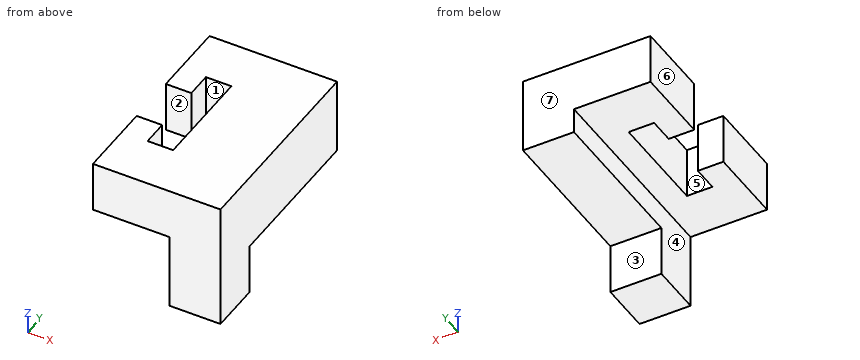
Autodesk Inventor part; units mm, degrees
ref_plane "YZ Plane" through (0, 0, 0) normal (1, 0, 0) x (0, 1, 0)
ref_plane "XZ Plane" through (0, 0, 0) normal (0, 1, 0) x (-1, 0, 0)
ref_plane "XY Plane" through (0, 0, 0) normal (0, 0, 1) x (1, 0, 0)
sketch "Náčrt1" plane through (0, 0, 0) normal (1, 0, 0) x (0, 1, 0)
  line L0 (0, 0) -> (0, -50)
  line L1 (0, -50) -> (80, -50)
  line L2 (80, -50) -> (80, 0)
  line L3 (80, 0) -> (0, 0)
  dimension "d0" = 50
  dimension "d1" = 80
extrude "Vysunutí1" add sketch "Náčrt1" along normal blind 50
sketch "Náčrt2" plane through (0, 0, -50) normal (0, 0, -1) x (-1, 0, 0)
  line L0 (-50, 0) -> (-50, 80)
  line L1 (-50, 0) -> (-50, 20)
  line L2 (-50, 20) -> (-30, 20)
  line L3 (-30, 20) -> (-30, 0)
  line L4 (0, 0) -> (-50, 0)
  line L5 (-30, 0) -> (-50, 0)
  line L6 (-50, 0) -> (-50, 80)
  line L7 (-50, 80) -> (-30, 80)
  line L8 (0, 80) -> (-50, 80)
  line L9 (-30, 80) -> (-30, 20)
  dimension "d4" = 20
  dimension "d5" = 20
  dimension "d6" = 20
extrude "Vysunutí2" cut sketch "Náčrt2" against normal blind 20 contours L0 L7 L9 L2
sketch "Náčrt3" plane through (0, 0, -50) normal (0, 0, -1) x (-1, 0, 0)
  line L0 (0, 80) -> (-50, 80)
  line L1 (0, 0) -> (0, 80)
  line L2 (0, 80) -> (0, 0)
  line L3 (0, 0) -> (-30, 0)
  line L4 (0, 0) -> (-50, 0)
  line L5 (-30, 0) -> (-30, 80)
  dimension "d9" = 30
extrude "Vysunutí3" cut sketch "Náčrt3" against normal blind 30
sketch "Náčrt4" plane through (0, 0, -20) normal (0, 0, -1) x (-1, 0, 0)
  line L0 (0, 80) -> (0, 0)
  line L1 (0, 40) -> (0, 30)
  line L2 (0, 30) -> (0, 50)
  line L3 (0, 50) -> (-10, 50)
  line L4 (0, 40) -> (-20, 40)
  line L5 (-20, 40) -> (-20, 60)
  line L6 (-20, 60) -> (-10, 60)
  line L7 (-10, 50) -> (-10, 60)
  line L8 (0, 30) -> (-10, 30)
  dimension "d12" = 10
  dimension "d13" = 20
  dimension "d14" = 10
  dimension "d15" = 20
  dimension "d16" = 20
  dimension "d17" = 10
extrude "Vysunutí4" cut sketch "Náčrt4" against normal blind 30
sketch "Náčrt5" plane through (0, 0, -20) normal (0, 0, -1) x (-1, 0, 0)
  line L0 (0, 40) -> (0, 0)
  line L1 (-20, 40) -> (-20, 60)
  line L2 (0, 40) -> (-20, 40)
  line L3 (-20, 40) -> (-20, 20)
  line L4 (-20, 20) -> (-10, 20)
  line L5 (-10, 20) -> (-10, 30)
  line L6 (-10, 30) -> (0, 30)
  line L7 (0, 40) -> (0, 0)
  line L8 (0, 30) -> (0, 40)
  dimension "d20" = 20
  dimension "d21" = 10
  dimension "d22" = 10
extrude "Vysunutí5" cut sketch "Náčrt5" against normal blind 30
properties part number "Martin-Probst-26673_obrazek_2"
Read the model definition and answer for the solid it produces. Units are mm, in the model's axes. Face numbers are marked on the shaded views. A direction names the side the tool comes from. Coordinates: 2 decimals unless noted, no trailing zeros. Write each loop counter-clockwise with the first axis right and the second up, starting at its lowest first coordinate (ties: lowest second). Pieces come first, ordered by that corner, then holes. Notation, with made-up numbers: M 52,0.5 L 91,0.5 A29 ccw 91,29.5 Z; hole C 70,-29.75 d11. An arc over 180 degrees is marked long. Use a Markdown table: item, result.
Q1. The part is cut by section B-B, the plane y = 58.5. Write down the section's boundary in (x, z), then the cut area to 3 significant figures.
Answer block:
| item | result |
|---|---|
| outline | M 0,-20 L 10,-20 L 10,0 L 0,0 Z; M 20,-20 L 30,-20 L 30,-30 L 50,-30 L 50,0 L 20,0 Z |
| area | 1,000 mm2 |
Q2. Determine the mould class of the marked faces 5, 6 and 7 for opening direction Y: released by +Y, released by -Y, zero draft, split by the parting line, or undercut.
Answer block:
| item | result |
|---|---|
| face 5 | undercut |
| face 6 | zero draft |
| face 7 | released by +Y |
Q3. The part is cut by section D-D, the plane y = 10.5. Write down the section's boundary in (x, z).
Answer block:
| item | result |
|---|---|
| outline | M 0,-20 L 30,-20 L 30,-50 L 50,-50 L 50,0 L 0,0 Z |
Q4. The part is cut by section A-A, the plane x = 15.5. Write down the section's boundary in (y, z).
Answer block:
| item | result |
|---|---|
| outline | M 0,-20 L 20,-20 L 20,0 L 0,0 Z; M 60,-20 L 80,-20 L 80,0 L 60,0 Z |
Q5. The part is cut by section C-C, the plane z = -11.5. Write down the section's boundary in (x, y).
Answer block:
| item | result |
|---|---|
| outline | M 0,0 L 50,0 L 50,80 L 0,80 L 0,50 L 10,50 L 10,60 L 20,60 L 20,20 L 10,20 L 10,30 L 0,30 Z |
Q6. Straight lines are drawn through the part: L1, parallel to Y at x = 7.5, z = -3.5; L2, parallel to Y at x = 48, z = -36.5; L3, parallel to X at y = 13, z = -43.5. For each, find the intervals that lie inside material, in ascending order. Write a range as [from, to].
Answer block:
| item | result |
|---|---|
| L1 | y = [0, 30], [50, 80] |
| L2 | y = [0, 20] |
| L3 | x = [30, 50] |
Q7. Each of these flat-tipped pins is pushed along its axis until it touches: pin 1 Ø16 at (y, z) = (43, -10.5) entering from -X; pin 2 Ø9 at (y, z) = (35, -31) entering from -X; pin 3 Ø10 at (x, z) = (41.5, -38) entering from +Y; pin 4 Ø10 at (x, y) = (37.5, 47) entering from -Z. Where does it stop, or does it pass through?
Answer block:
| item | result |
|---|---|
| pin 1 | stops at x = 0 |
| pin 2 | stops at x = 30 |
| pin 3 | stops at y = 20 |
| pin 4 | stops at z = -30 |
Q8. Which of the six approach directions +Z, -Z, +X, -X, +Y, -Y give full straight-line access (tool end or side, diameter ignored) to the marked faces 1, 2, 3 and 4?
Answer block:
| item | result |
|---|---|
| face 1 | +Z, -Z |
| face 2 | +Z, -Z, -X |
| face 3 | -Z, +X, -X, +Y |
| face 4 | -Z, -X, +Y, -Y |
